from build123d import *

# Parameters (mm, degrees)
FILLET1_R          = 1.5
SKETCH3_W          = 2
SKETCH3_H          = 2
CUT_EXTRUDE1_DEPTH = 62.42


with BuildPart() as part:
    # Sketch2 → Revolve1 (revolve)
    with BuildSketch(Plane.XY, mode=Mode.PRIVATE) as revolve1_sk:
        with BuildLine():
            Line((0, 25), (0, 10.65))
            Line((0, 10.65), (-67.42, 10.65))
            Line((-67.42, 10.65), (-67.42, 0))
            Line((-67.42, 0), (-70.42, 0))
            Line((-70.42, 0), (-70.42, 9.65))
            ThreePointArc((-70.42, 9.65), (-68.955533906, 13.185533906), (-65.42, 14.65))
            Line((-65.42, 14.65), (-3, 14.65))
            Line((-3, 14.65), (-3, 25))
            Line((-3, 25), (0, 25))
        make_face()
    revolve(revolve1_sk.sketch.rotate(Axis((-556.896186161, 0, 0), (1, 0, 0)), 90), axis=Axis((-556.896186161, 0, 0), (1, 0, 0)))

    # Fillet1
    fillet1_edges = [part.edges().sort_by_distance(p)[0] for p in [
        (0, 0, -25),
        (-3, 0, -25),
    ]]
    fillet(fillet1_edges, radius=FILLET1_R - 0.0001)  # a hair under: the kernel refuses the full size

    # Sketch3 → Cut-Extrude1 (cut)
    with BuildSketch(Plane.ZY.offset(3)):
        Polygon((2.6341252, 15.450463157), (2.172893459, 13.504373416), (4.1189832, 13.043141675), (4.580214941, 14.989231416), align=None)
        with Locations((0, 14.641465)):
            Rectangle(SKETCH3_W, SKETCH3_H)
        Polygon((6.126244029, 14.426522847), (5.228645668, 12.639257566), (7.015910949, 11.741659206), (7.913509309, 13.528924486), align=None)
        Polygon((9.288095456, 12.624844955), (8.002520237, 11.092756069), (9.534609123, 9.80718085), (10.820184342, 11.339269736), align=None)
        Polygon((11.949223253, 10.142558404), (10.344976868, 8.948241221), (11.539294051, 7.343994835), (13.143540437, 8.538312019), align=None)
        Polygon((13.966165332, 7.113483905), (12.129733118, 6.321324373), (12.92189265, 4.484892159), (14.758324864, 5.277051691), align=None)
        Polygon((15.230187823, 3.700919646), (13.260572317, 3.353623291), (13.607868672, 1.384007785), (15.577484178, 1.73130414), align=None)
        Polygon((15.673146946, 0.088837852), (13.676530629, 0.20512751), (13.560240971, -1.791488807), (15.556857288, -1.907778465), align=None)
        Polygon((15.27116266, -3.528033214), (13.355183635, -2.954426749), (12.78157717, -4.870405773), (14.697556195, -5.444012239), align=None)
        Polygon((14.045906042, -6.954707096), (12.313855235, -5.954707096), (11.313855235, -7.686757904), (13.045906042, -8.686757904), align=None)
        Polygon((12.063430994, -10.006450919), (10.608683711, -8.633967643), (9.236200436, -10.088714926), (10.690947719, -11.461198202), align=None)
        Polygon((9.430613259, -12.518744382), (8.331595303, -10.847768759), (6.66061968, -11.946786715), (7.759637636, -13.617762338), align=None)
        Polygon((6.289388722, -14.356149095), (5.605348435, -12.476763854), (3.725963194, -13.160804141), (4.41000348, -15.040189382), align=None)
        Polygon((2.809101611, -15.419610095), (2.576915783, -13.43313338), (0.590439067, -13.665319208), (0.822624895, -15.651795923), align=None)
        Polygon((-0.822624895, -15.651795923), (-0.590439067, -13.665319208), (-2.576915783, -13.43313338), (-2.809101611, -15.419610095), align=None)
        Polygon((-4.41000348, -15.040189382), (-3.725963194, -13.160804141), (-5.605348435, -12.476763854), (-6.289388722, -14.356149095), align=None)
        Polygon((-7.759637636, -13.617762338), (-6.66061968, -11.946786715), (-8.331595303, -10.847768759), (-9.430613259, -12.518744382), align=None)
        Polygon((-10.690947719, -11.461198202), (-9.236200436, -10.088714926), (-10.608683711, -8.633967643), (-12.063430994, -10.006450919), align=None)
        Polygon((-13.045906042, -8.686757904), (-11.313855235, -7.686757904), (-12.313855235, -5.954707096), (-14.045906042, -6.954707096), align=None)
        Polygon((-14.697556195, -5.444012239), (-12.78157717, -4.870405773), (-13.355183635, -2.954426749), (-15.27116266, -3.528033214), align=None)
        Polygon((-15.556857288, -1.907778465), (-13.560240971, -1.791488807), (-13.676530629, 0.20512751), (-15.673146946, 0.088837852), align=None)
        Polygon((-15.577484178, 1.73130414), (-13.607868672, 1.384007785), (-13.260572317, 3.353623291), (-15.230187823, 3.700919646), align=None)
        Polygon((-14.758324864, 5.277051691), (-12.92189265, 4.484892159), (-12.129733118, 6.321324373), (-13.966165332, 7.113483905), align=None)
        Polygon((-13.143540437, 8.538312019), (-11.539294051, 7.343994835), (-10.344976868, 8.948241221), (-11.949223253, 10.142558404), align=None)
        Polygon((-10.820184342, 11.339269736), (-9.534609123, 9.80718085), (-8.002520237, 11.092756069), (-9.288095456, 12.624844955), align=None)
        Polygon((-7.913509309, 13.528924486), (-7.015910949, 11.741659206), (-5.228645668, 12.639257566), (-6.126244029, 14.426522847), align=None)
        Polygon((-4.580214941, 14.989231416), (-4.1189832, 13.043141675), (-2.172893459, 13.504373416), (-2.6341252, 15.450463157), align=None)
    extrude(amount=CUT_EXTRUDE1_DEPTH, mode=Mode.SUBTRACT)


solid = part.part
The model under review builds one solid part; all positions refer to its coordinate system, in mm. A direction names the side the tool comes from. Coordinates: 2 decimals unless noted, no trailing zeros. Answer in a Markdown table with one row per item.
(1) The part is to be moulded in two halves that separate along Z. For faces 3 (the flat face through (0, 5, 10)), 4 (the flat face through (-33.773, -11.405, -7.484)), say which applies: +Z half, -Z half, draft (parallel to the pull), parting line (faces both ways), or undercut.
Answers:
| item | result |
|---|---|
| face 3 | draft |
| face 4 | undercut |
(2) Machinability: for faces 1 (the flat face through (-67.42, 0, 0)), 2 (the flat face through (-33.773, 8.135, -10.95)), which of the approach directions +Z, -Z, +X, -X, +Y, -Y give a long, thin tool a straight path to every point of the face, cutting with its end or side? Answer none if there is none.
Answers:
| item | result |
|---|---|
| face 1 | +X |
| face 2 | none |
(3) Wall thickness on line 1 along Z through (x, y) = (-38, -9); line 2 along X through (y, z) = (-2.5, 6); line 3 along X through (y, z) = (19.5, -13): over which ranges is each line inside the solid? List them lowest first.
Answers:
| item | result |
|---|---|
| line 1 | -11.56 to -11, -10.26 to -5.69, 5.69 to 10.26, 11 to 11.56 |
| line 2 | -70.42 to -67.42 |
| line 3 | -3 to 0 |
(4) Insertion check: pin 1 (5 mm diameter, centred on x = -34.5, y = -0.5, fed in from -Z); pin 2 (1.6 mm diameter, centred on x = -23, z = 0.5, fed in from +Y); pin 3 (5 mm diameter, centred on x = -32.5, z = -2, fed in from -Y). Each pin has a flat end and moves straight along its axis. Give the tip position at first contact, or say it passes through.
Answers:
| item | result |
|---|---|
| pin 1 | z = -14.65 |
| pin 2 | y = 14.62 |
| pin 3 | y = -14.65 |
